```python
from build123d import *

# Parameters (mm, degrees)
EXTRUDE_1_DEPTH          = 65
SKETCH_3_R               = 2
CUT_EXTRUDE_2_DEPTH      = 136.321005452
SKETCH_4_W               = 30
SKETCH_4_H               = 22
EXTRUDE_2_DEPTH          = 5
CUT_EXTRUDE_4_DEPTH      = 123.556209621
CUT_EXTRUDE_4_DEPTH_BACK = 123.556209621
SKETCH_9_R               = 1.45
SKETCH_10_W              = 20
SKETCH_10_H              = 22
SKETCH_10_W_2            = 5
SKETCH_10_H_2            = 8
EXTRUDE_6_DEPTH          = 11


with BuildPart() as part:
    # 草圖1 → 填料-伸長1 (new body)
    with BuildSketch(Plane.XY):
        Polygon((-26.364407373, 0.778312538), (-21.364407373, 0.778312538), (-21.364407373, -22.221687462), (-34.864407373, -22.221687462), (-34.864407373, -44.221687462), (67.135592627, -44.221687462), (67.135592627, -22.221687462), (53.635592627, -22.221687462), (53.635592627, 0.778312538), (58.635592627, 0.778312538), (58.635592627, -17.221687462), (70.135592627, -17.221687462), (70.135592627, -49.221687462), (-37.864407373, -49.221687462), (-37.864407373, -17.221687462), (-26.364407373, -17.221687462), align=None)
    extrude(amount=EXTRUDE_1_DEPTH)

    # 草圖3 → 除料-伸長2 (cut, through all)
    with BuildSketch(Plane.ZY.offset(37.864407373)):
        with Locations((43.545745688, -33.221687462)):
            Circle(SKETCH_3_R)
    extrude(amount=-CUT_EXTRUDE_2_DEPTH, mode=Mode.SUBTRACT)

    # 草圖4 → 填料-伸長2 (add)
    with BuildSketch(Plane(origin=(0, 0, 0), x_dir=(-1, 0, 0), z_dir=(0, 0, -1))):
        with Locations((-27.135592627, -33.221687462)):
            Rectangle(SKETCH_4_W, SKETCH_4_H)
    extrude(amount=-EXTRUDE_2_DEPTH)

    # 草圖9 → 除料-伸長4 (cut, two sides: drawn at the far end of the back side and taken through both)
    with BuildSketch(Plane(origin=(-21.364407373, 0, 0), x_dir=(0, 0, -1), z_dir=(1, 0, 0)).offset(-CUT_EXTRUDE_4_DEPTH_BACK)):
        with Locations(Location((-31.5, -4.221687462, 0), (0, 0, 90))):
            Circle(SKETCH_9_R)
        with Locations(Location((-16.5, -4.221687462, 0), (0, 0, 90))):
            Circle(SKETCH_9_R)
    extrude(amount=CUT_EXTRUDE_4_DEPTH + CUT_EXTRUDE_4_DEPTH_BACK, mode=Mode.SUBTRACT)

    # 草圖10 → 填料-伸長6 (add)
    # profile 1 of 2: a face of its own
    with BuildSketch(Plane.XY.offset(65)):
        with Locations((-24.864407373, -33.221687462)):
            Rectangle(SKETCH_10_W, SKETCH_10_H)
        with Locations((-23.864407373, -33.221687462)):
            Rectangle(SKETCH_10_W_2, SKETCH_10_H_2, mode=Mode.SUBTRACT)
    # profile 2 of 2: a face of its own
    with BuildSketch(Plane.XY.offset(65)):
        with Locations((57.135592627, -33.221687462)):
            Rectangle(SKETCH_10_W, SKETCH_10_H)
        with Locations((56.135592627, -33.221687462)):
            Rectangle(SKETCH_10_W_2, SKETCH_10_H_2, mode=Mode.SUBTRACT)
    extrude(amount=-EXTRUDE_6_DEPTH)


solid = part.part
```
CAD build for the part. Positions are in the model's coordinates, mm. A direction names the side the tool comes from. Coordinates: 2 decimals unless noted, no trailing zeros. Order: outer loops, then holes, each group sorted by start corner. A loop starts at its lowest first (then second) coordinate and runs counter-clockwise, first axis right, second up. Notation, with made-up numbers: (42.5, 69.5) - (100.5, 69.5) arc R21 cw to (100.5, 104.5) - close; hole circle Ø4 at (52.25, -21.75). An arc over 180 degrees is marked (long way). Answer in a Markdown table with one row per item.
1. Slice it at B-B, the plane z = 31.5. List the corners of the cut face in (x, y), then the cut area to 3 significant figures.
Answer:
| item | result |
|---|---|
| outline | (-37.86, -49.22) - (70.14, -49.22) - (70.14, -17.22) - (58.64, -17.22) - (58.64, -5.67) - (53.64, -5.67) - (53.64, -22.22) - (67.14, -22.22) - (67.14, -44.22) - (-34.86, -44.22) - (-34.86, -22.22) - (-21.36, -22.22) - (-21.36, -5.67) - (-26.36, -5.67) - (-26.36, -17.22) - (-37.86, -17.22) - close; (-26.36, -2.77) - (-21.36, -2.77) - (-21.36, 0.78) - (-26.36, 0.78) - close; (53.64, -2.77) - (58.64, -2.77) - (58.64, 0.78) - (53.64, 0.78) - close |
| area | 988 mm² |
2. Slice it at D-D, the plane z = 11.5. List the corners of the cut face in (x, y), then the cut area to 3 significant figures.
Answer:
| item | result |
|---|---|
| outline | (-37.86, -49.22) - (70.14, -49.22) - (70.14, -17.22) - (58.64, -17.22) - (58.64, 0.78) - (53.64, 0.78) - (53.64, -22.22) - (67.14, -22.22) - (67.14, -44.22) - (-34.86, -44.22) - (-34.86, -22.22) - (-21.36, -22.22) - (-21.36, 0.78) - (-26.36, 0.78) - (-26.36, -17.22) - (-37.86, -17.22) - close |
| area | 1,020 mm² |
3. Slice it at C-C, the plane x = -18. List the corners of the cut face in (y, z), then the cut area to 3 significant figures.
Answer:
| item | result |
|---|---|
| outline | (-49.22, 0) - (-44.22, 0) - (-44.22, 54) - (-22.22, 54) - (-22.22, 65) - (-49.22, 65) - close |
| area | 567 mm² |
4. Slice it at A-A, the plane y = -39. List the corners of the cut face in (x, z), then the cut area to 3 significant figures.
Answer:
| item | result |
|---|---|
| outline | (-37.86, 0) - (-34.86, 0) - (-34.86, 54) - (-14.86, 54) - (-14.86, 65) - (-37.86, 65) - close; (12.14, 0) - (42.14, 0) - (42.14, 5) - (12.14, 5) - close; (47.14, 54) - (67.14, 54) - (67.14, 0) - (70.14, 0) - (70.14, 65) - (47.14, 65) - close |
| area | 980 mm² |
5. Pull direction Y, two halves, no side cores. Call faces 5 (the face through (-24, 0.778, 32)), 6 (the face through (47.136, -33, 60)), 7 (the face through (17, -49.222, 32)), 8 (the face through (-24, -29.222, 60)): +Y half, -Y half, draft (parallel to the pull), parting line (faces both ways), or undercut.
Answer:
| item | result |
|---|---|
| face 5 | +Y half |
| face 6 | draft |
| face 7 | -Y half |
| face 8 | undercut |
6. Drill centre lines: L1, parallel to X at y = -38, z = 4; L2, parallel to X at y = -18, z = 40; L3, parallel to X at y = -43.5, z = 51. Where is each one in solid material? Low to high. Write a range as from..to.
Answer:
| item | result |
|---|---|
| L1 | -37.86..-34.86, 12.14..42.14, 67.14..70.14 |
| L2 | -37.86..-21.36, 53.64..70.14 |
| L3 | -37.86..-34.86, 67.14..70.14 |
7. 3-axis set-ups, long thin cutter, end or side, ignore diameter. For faces 1 (the face through (59, -33, 54)), 2 (the face through (27, -22.222, 2)), 3 (the face through (58.636, -33, 60)), 4 (the face through (27, -33, 5)): which of +Z, -Z, +X, -X, +Y, -Y reach the whole face in a straight line?
Answer:
| item | result |
|---|---|
| face 1 | -Z |
| face 2 | +Z, -Z, +Y |
| face 3 | +Z, -Z |
| face 4 | +Z, +Y |
8. Flat gauge pins, fed straight in: P1, Ø20, axis at y = -12, z = 43.5, coming from the +X side; P2, Ø12, axis at y = -6, z = 38.5, coming from the +X side; P3, Ø1.5, axis at x = 20.5, z = 47, coming from the +Y side; P4, Ø2, axis at x = 49.5, z = 58, coming from the +Y side. Where does each tip first touch, or does it go through?
Answer:
| item | result |
|---|---|
| P1 | x = 70.14 |
| P2 | x = 58.64 |
| P3 | y = -44.22 |
| P4 | y = -22.22 |
